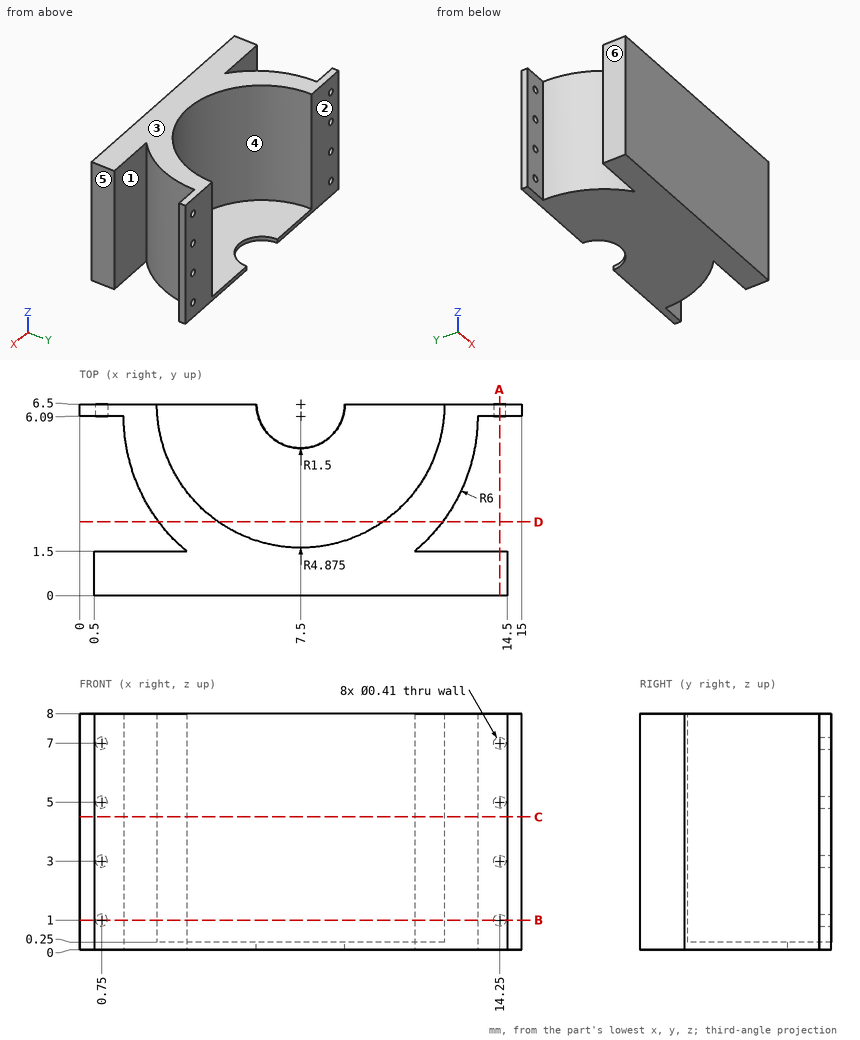
The drawing under review shows one solid part. Ordinate dimensions are in mm from its lowest x, y, z. A direction names the side the tool comes from. Coordinates: 2 decimals unless noted, no trailing zeros. Order: outer loops, then holes, each group sorted by start corner. A loop starts at its lowest first (then second) coordinate and runs counter-clockwise, first axis right, second up. Notation, with made-up numbers: M -11.5,26 L 39.5,26 A17 ccw 39.5,56 Z; hole C -24,77 d4. An arc over 180 degrees is marked long. Use a Markdown table: item, result.
(1) Add section D-D (y = 2.5). Give the boundary of the cut face in (x, z).
Worked answers:
| item | result |
|---|---|
| outline | M 2.69,0 L 12.31,0 L 12.31,8 L 10.29,8 L 10.29,0.25 L 4.71,0.25 L 4.71,8 L 2.69,8 Z |
(2) Add section A-A (x = 14.25). Give the boundary of the cut face in (y, z) (3 decimals), then the cut area to 3 significant figures.
Worked answers:
| item | result |
|---|---|
| outline | M 0,0 L 1.5,0 L 1.5,8 L 0,8 Z; M 6.09,0 L 6.5,0 L 6.5,0.795 L 6.09,0.795 Z; M 6.09,1.205 L 6.5,1.205 L 6.5,2.795 L 6.09,2.795 Z; M 6.09,3.205 L 6.5,3.205 L 6.5,4.795 L 6.09,4.795 Z; M 6.09,5.205 L 6.5,5.205 L 6.5,6.795 L 6.09,6.795 Z; M 6.09,7.205 L 6.5,7.205 L 6.5,8 L 6.09,8 Z |
| area | 14.6 mm2 |
(3) Add section C-C (z = 4.5). Give the boundary of the cut face in (x, y) (3 decimals), then the cut area to 3 significant figures.
Worked answers:
| item | result |
|---|---|
| outline | M 0,6.09 L 1.5,6.09 A6 ccw 3.636,1.5 L 0.5,1.5 L 0.5,0 L 14.5,0 L 14.5,1.5 L 11.364,1.5 A6 ccw 13.5,6.09 L 15,6.09 L 15,6.5 L 12.375,6.5 A4.875 cw 2.625,6.5 L 0,6.5 Z |
| area | 38.9 mm2 |
(4) Add section B-B (z = 1). Give the boundary of the cut face in (x, y) (3 decimals), then the cut area to 3 significant figures.
Worked answers:
| item | result |
|---|---|
| outline | M 0,6.09 L 0.545,6.09 L 0.545,6.5 L 0,6.5 Z; M 0.5,0 L 14.5,0 L 14.5,1.5 L 11.364,1.5 A6 ccw 13.5,6.09 L 14.045,6.09 L 14.045,6.5 L 12.375,6.5 A4.875 cw 2.625,6.5 L 0.955,6.5 L 0.955,6.09 L 1.5,6.09 A6 ccw 3.636,1.5 L 0.5,1.5 Z; M 14.455,6.09 L 15,6.09 L 15,6.5 L 14.455,6.5 Z |
| area | 38.6 mm2 |
(5) Wall thickness on probe 1 along Z at (x, y) = (14.25, 6.25) (3 decimals); probe 2 along Y at (x, z) = (14, 3.25); probe 3 along X at (y, z) = (0.5, 6.5): over which ranges is each line inside the solid? List them lowest first.
Worked answers:
| item | result |
|---|---|
| probe 1 | z = 0 to 0.795, 1.205 to 2.795, 3.205 to 4.795, 5.205 to 6.795, 7.205 to 8 |
| probe 2 | y = 0 to 1.5, 6.09 to 6.5 |
| probe 3 | x = 0.5 to 14.5 |
(6) Draft analysis for pull direction Y (two halves, no side actions). For the marked faces 1, 2 and 3, state which applies: released by +Y, released by -Y, zero draft, split by the parting line, or undercut.
Worked answers:
| item | result |
|---|---|
| face 1 | undercut |
| face 2 | released by +Y |
| face 3 | zero draft |
(7) For P1, Ø1.2, axis at y = 1, z = 4.5, coming from the -X side; P2, Ø2, axis at y = 4.5, z = 7, coming from the +X side, all flat-tipped, find the tip position at first contact; note any pin that passes through.
Worked answers:
| item | result |
|---|---|
| P1 | stops at x = 0.5 |
| P2 | stops at x = 13.47 |
(8) For the marked faces 4, 5 and 6, list the 3-axis set-ups (+Z, -Z, +X, -X, +Y, -Y) from which the entire face can be reached by the end or side of a thin tool; tool diameter is ignored.
Worked answers:
| item | result |
|---|---|
| face 4 | +Z, +Y |
| face 5 | +Z, -Z, +X, -Y |
| face 6 | +Z, -Z, -X, -Y |
